Autodesk Inventor part; units mm, degrees
ref_plane "YZ Plane" through (0, 0, 0) normal (1, 0, 0) x (0, 1, 0)
ref_plane "XZ Plane" through (0, 0, 0) normal (0, 1, 0) x (-1, 0, 0)
ref_plane "XY Plane" through (0, 0, 0) normal (0, 0, 1) x (1, 0, 0)
sketch "スケッチ1" plane through (0, 0, 0) normal (0, 0, 1) x (1, 0, 0)
  line L0 (0, 0) -> (-2.7189, -1.2679) construction
  line L1 (0, 0) -> (0, -26) construction
  arc A0 (8.8407, -4.1114) -> (-9.5086, -2.1563) centre (0, 0) ccw
  arc A1 (-3.901, -26.8846) -> (4, -26) centre (0, -26) ccw
  arc A2 (8.8407, -4.1114) -> (4, -26) centre (55.9076, -26) ccw
  line L2 (-9.5086, -2.1563) -> (-3.901, -26.8846)
  line L3 (0, -26) -> (4, -26) construction
  circle A3 centre (0, 0) radius 8 construction
  point P0 (8, 0)
  point P1 (5.6569, 5.6569)
  point P2 (0, 8)
  point P3 (-5.6569, 5.6569)
  point P4 (-8, 0)
  point P5 (-5.6569, -5.6569)
  point P6 (0, -8)
  point P7 (5.6569, -5.6569)
  point P8 (0, -26)
  dimension "d38" = 16
  dimension "d2" = 3
  dimension "d4" = 26
  dimension "d6" = 9.75
  dimension "d7" = 4
  dimension "d11" = 360
  dimension "d37" = 65
extrude "押し出し1" add sketch "スケッチ1" along normal blind 3
hole "穴1" at (8, 0, 0) at (5.6569, 5.6569, 0) at (0, 8, 0) at (-5.6569, 5.6569, 0) at (-8, 0, 0) at (-5.6569, -5.6569, 0) at (0, -8, 0) at (5.6569, -5.6569, 0) direction (0, 0, 1) diameter 2 end through all
hole "穴2" at (0, -26, 0) direction (0, 0, 1) diameter 3 end through all
sketch "スケッチ2" plane through (0, 0, 0) normal (0, 0, -1) x (-1, 0, 0)
  circle A0 centre (0, 0) radius 4
  dimension "d30" = 8
extrude "押し出し2" cut sketch "スケッチ2" against normal blind 2
sketch "スケッチ3" plane through (0, 0, 3) normal (0, 0, 1) x (1, 0, 0)
  circle A0 centre (-2.7189, -1.2679) radius 2
  point P0 (0, 0)
  dimension "d33" = 4
extrude "押し出し3" add sketch "スケッチ3" along normal blind 3
properties part number "COXA_ROLL_SERVO-OUTPUT"
Model file for the job. Use its own axes, mm. A direction names the side the tool comes from. Coordinates: 2 decimals unless noted, no trailing zeros. Order: outer loops, then holes, each group sorted by start corner. A loop starts at its lowest first (then second) coordinate and runs counter-clockwise, first axis right, second up. Notation, with made-up numbers: (44, -35) -> (68, -35) arc R24 cw to (68, 4) -> close; hole circle Ø8 at (33.5, -35). An arc over 180 degrees is marked (long way). Answer as a JSON object with one key per item and string values. Group by question number.
1) Pull direction X, two halves, no side cores. Call faces 1 (the face through (6.265, -6.45, 1.521)), 2 (the face through (0, -10, 3)), 3 (the face through (5.2, -14.9, 1.5)): +X half, -X half, draft (parallel to the pull), parting line (faces both ways), or undercut.
2) Cut at C-C, the plane y = 0. Write the cut outline in (x, z), then the cut area to 3 significant figures.
3) Cut at A-A, the plane x = 0. Write the cut outline in (y, z), then the cut area to 4 significant figures.
4) Flat gauge pins, fed straight in: pin 1 (1.8 mm diameter, centred on x = 0, y = -8, fed in from -Z); pin 2 (1.5 mm diameter, centred on y = -1.5, z = 1.5, fed in from -X); pin 3 (2.5 mm diameter, centred on x = -8, y = 0, fed in from +Z); pin 4 (2.5 mm diameter, centred on x = -1, y = 0.5, fed in from -Z). Where does each tip first touch, or does it go through?
5) Cut at B-B, the plane y = 8. Write the cut outline in (x, z), then the cut area to 3 significant figures.
6) Cut at D-D, the plane x = 8. Write the cut outline in (y, z), then the cut area to 3 significant figures.
7) Which spindle directions (+Z, -Z, +X, -X, +Y, -Y) get a long thin tool onto all of the face, cutting with end or side? Do faces 4 (the face through (0.867, -3.905, 0.986)), 5 (the face through (-0.81, -1.87, 4.48)), 6 (the face through (0.526, -29.965, 1.479)). Say none if no direction does.
8) Drill centre lines: L1, parallel to Y at x = 0, z = 0.95; L2, parallel to Z at x = -5.75, y = -16; L3, parallel to Y at x = 2.75, z = 0.4. Where is each one in solid material? Low to high.
Check values:
{
 "1": {"face 1": "undercut", "face 2": "draft", "face 3": "+X half"},
 "2": {"outline": "(-9.75, 0) -> (-9, 0) -> (-9, 3) -> (-9.75, 3) -> close; (-7, 0) -> (-4, 0) -> (-4, 2) -> (4, 2) -> (4, 0) -> (7, 0) -> (7, 3) -> (-1.17, 3) -> (-1.17, 6) -> (-4.27, 6) -> (-4.27, 3) -> (-7, 3) -> close; (9, 0) -> (9.75, 0) -> (9.75, 3) -> (9, 3) -> close", "area": "39.8 mm²"},
 "3": {"outline": "(-30, 0) -> (-27.5, 0) -> (-27.5, 3) -> (-30, 3) -> close; (-24.5, 0) -> (-9, 0) -> (-9, 3) -> (-24.5, 3) -> close; (-7, 0) -> (-4, 0) -> (-4, 2) -> (4, 2) -> (4, 0) -> (7, 0) -> (7, 3) -> (-7, 3) -> close; (9, 0) -> (9.75, 0) -> (9.75, 3) -> (9, 3) -> close", "area": "82.25 mm²"},
 "4": {"pin 1": "passes through", "pin 2": "stops at x = -9.72", "pin 3": "stops at z = 3", "pin 4": "stops at z = 2"},
 "5": {"outline": "(-5.57, 0) -> (-1, 0) -> (-1, 3) -> (-5.57, 3) -> close; (1, 0) -> (5.57, 0) -> (5.57, 3) -> (1, 3) -> close", "area": "27.4 mm²"},
 "6": {"outline": "(-6.02, 0) -> (-1, 0) -> (-1, 3) -> (-6.02, 3) -> close; (1, 0) -> (5.57, 0) -> (5.57, 3) -> (1, 3) -> close", "area": "28.8 mm²"},
 "7": {"face 4": "-Z", "face 5": "+Z", "face 6": "+Z, -Z, -Y"},
 "8": {"L1": "y = -30 to -27.5, -24.5 to -9, -7 to -4, 4 to 7, 9 to 9.75", "L2": "z = 0 to 3", "L3": "y = -28.9 to -2.9, 2.9 to 9.35"}
}
